Geometry: final body of the model. Coordinates: model frame, mm. Face numbers are marked on the shaded views. Give positions to 0.01 mm unless a question says otherwise; leave off trailing zeros. Write each loop counter-clockwise with the first axis right and the second up, starting at its lowest first coordinate (ties: lowest second). Pieces come first, ordered by that corner, then holes. Notation, with made-up numbers: (-7.75, 24) -> (24.25, 24) arc R15 ccw to (24.25, 48) -> close; hole circle Ø6 at (20, 36). An arc over 180 degrees is marked (long way). Use CSV: the item, a comma, the result in double quotes. Start each with the question number.
1) Section A-A (y = 0). Output: boundary loops of the cut face in (x, z).
2) Section B-B (x = 0). Output: boundary loops of the cut face in (y, z).
3) Draft query along X for the marked faces 1, 2 and 3. Return one class per face: pulls with the +X half, pulls with the -X half, needs draft (parallel to the pull), parting line crosses it, or undercut.
4) Contact query for flat-ended pins moving along their axis: P1, Ø1, axis at y = 64, z = 1, coming from the -X side; P2, Ø1, axis at y = 14, z = 1, coming from the +X side; P3, Ø1.6, axis at y = -69, z = 1, coming from the -X side; P4, Ø1.5, axis at x = 59, y = 38, coming from the -Z side. Output: stop coordinate, or through.
5) Material intervals for line 1 (Y direction, x = 0, z = 1.45); line 2 (Y direction, x = 0, z = 3.6); line 3 (Y direction, x = 11.5, z = 2.05), sorted ascending. Write a range as [from, to].
6) Section C-C (z = 3.8). Output: boundary loops of the cut face in (x, y).
7) Section D-D (y = -52.5). Output: boundary loops of the cut face in (x, z), plus the area to 3 significant figures.
```python
from build123d import *

# Parameters (mm, degrees)
SKETCH_1_R               = 87.5
EXTRUDE_1_DEPTH          = 5
SKETCH_7_W               = 16.5
SKETCH_7_H               = 3
CUT_EXTRUDE_3_DEPTH      = 10
PATTERN_CIRCULAR_1_COUNT = 2
SKETCH_8_W               = 16.1
SKETCH_8_H               = 30
CUT_EXTRUDE_4_DEPTH      = 2
PATTERN_CIRCULAR_2_COUNT = 2
SKETCH_9_R               = 9.25
CUT_EXTRUDE_5_DEPTH      = 2.5
SKETCH_10_R              = 12.6
CUT_EXTRUDE_6_DEPTH      = 2.5


with BuildPart() as part:
    # 草图1 → 凸台-拉伸1 (new body)
    with BuildSketch(Plane.XY):
        Circle(SKETCH_1_R)
    extrude(amount=EXTRUDE_1_DEPTH)

    # 草图7 → 切除-拉伸3 (cut)
    with BuildSketch(Plane(origin=(0, 0, 0), x_dir=(-1, 0, 0), z_dir=(0, 0, -1))):
        with Locations((0, 81)):
            Rectangle(SKETCH_7_W, SKETCH_7_H)
    cut_extrude_3 = extrude(amount=-CUT_EXTRUDE_3_DEPTH, mode=Mode.SUBTRACT)

    # 阵列(圆周)1: 切除-拉伸3 ×2 about axis
    pattern_circular_1_axis = Axis((0, 0, 0), (0, 0, 1))
    for i in range(1, PATTERN_CIRCULAR_1_COUNT):
        add(cut_extrude_3.rotate(pattern_circular_1_axis, i * 360 / PATTERN_CIRCULAR_1_COUNT), mode=Mode.SUBTRACT)

    # 草图8 → 切除-拉伸4 (cut)
    with BuildSketch(Plane(origin=(0, 0, 0), x_dir=(-1, 0, 0), z_dir=(0, 0, -1))):
        with Locations((0, 64.5)):
            Rectangle(SKETCH_8_W, SKETCH_8_H)
    cut_extrude_4 = extrude(amount=-CUT_EXTRUDE_4_DEPTH, mode=Mode.SUBTRACT)

    # 阵列(圆周)2: 切除-拉伸4 ×2 about axis
    pattern_circular_2_axis = Axis((0, 0, 0), (0, 0, 1))
    for i in range(1, PATTERN_CIRCULAR_2_COUNT):
        add(cut_extrude_4.rotate(pattern_circular_2_axis, i * 360 / PATTERN_CIRCULAR_2_COUNT), mode=Mode.SUBTRACT)

    # 草图9 → 切除-拉伸5 (cut)
    with BuildSketch(Plane.XY.offset(5)):
        Circle(SKETCH_9_R)
    extrude(amount=-CUT_EXTRUDE_5_DEPTH, mode=Mode.SUBTRACT)

    # 草图10 → 切除-拉伸6 (cut)
    with BuildSketch(Plane(origin=(0, 0, 0), x_dir=(-1, 0, 0), z_dir=(0, 0, -1))):
        Circle(SKETCH_10_R)
    extrude(amount=-CUT_EXTRUDE_6_DEPTH, mode=Mode.SUBTRACT)


solid = part.part
```
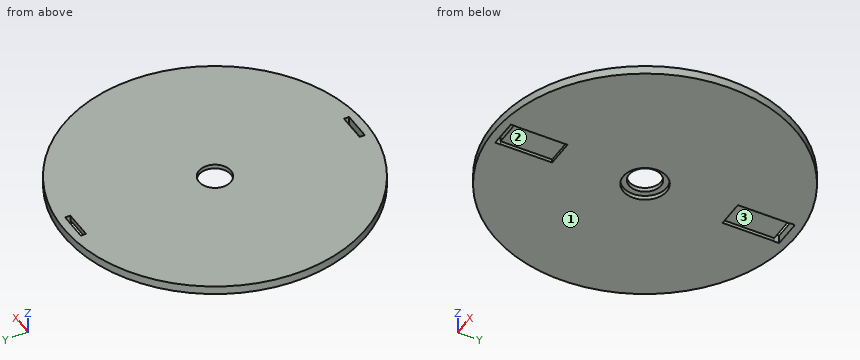
Answers follow:
1,outline,"(-87.5, 0) -> (-12.6, 0) -> (-12.6, 2.5) -> (-9.25, 2.5) -> (-9.25, 5) -> (-87.5, 5) -> close; (9.25, 2.5) -> (12.6, 2.5) -> (12.6, 0) -> (87.5, 0) -> (87.5, 5) -> (9.25, 5) -> close"
2,outline,"(-87.5, 0) -> (-82.5, 0) -> (-82.5, 5) -> (-87.5, 5) -> close; (-79.5, 2) -> (-49.5, 2) -> (-49.5, 0) -> (-12.6, 0) -> (-12.6, 2.5) -> (-9.25, 2.5) -> (-9.25, 5) -> (-79.5, 5) -> close; (9.25, 2.5) -> (12.6, 2.5) -> (12.6, 0) -> (49.5, 0) -> (49.5, 2) -> (79.5, 2) -> (79.5, 5) -> (9.25, 5) -> close; (82.5, 0) -> (87.5, 0) -> (87.5, 5) -> (82.5, 5) -> close"
3,face 1,"needs draft"
3,face 2,"undercut"
3,face 3,"undercut"
4,P1,"stops at x = -60.2"
4,P2,"stops at x = 86.45"
4,P3,"stops at x = -54.82"
4,P4,"stops at z = 0"
5,line 1,"y = [-87.5, -82.5], [-49.5, -12.6], [12.6, 49.5], [82.5, 87.5]"
5,line 2,"y = [-87.5, -82.5], [-79.5, -9.25], [9.25, 79.5], [82.5, 87.5]"
5,line 3,"y = [-86.74, -5.15], [5.15, 86.74]"
6,outline,"circle Ø175 at (0, 0); hole circle Ø18.5 at (0, 0); hole (-8.25, -82.5) -> (8.25, -82.5) -> (8.25, -79.5) -> (-8.25, -79.5) -> close; hole (-8.25, 79.5) -> (8.25, 79.5) -> (8.25, 82.5) -> (-8.25, 82.5) -> close"
7,outline,"(-70, 0) -> (-8.05, 0) -> (-8.05, 2) -> (8.05, 2) -> (8.05, 0) -> (70, 0) -> (70, 5) -> (-70, 5) -> close"
7,area,"668 mm^2"
